The listing builds one solid part. Answer for the finished solid, in the listing's coordinates (mm). Face numbers are marked on the shaded views. A direction names the side the tool comes from. Give positions to 0.01 mm unless a question says otherwise; leave off trailing zeros. Write each loop counter-clockwise with the first axis right and the second up, starting at its lowest first coordinate (ties: lowest second). Pieces come first, ordered by that corner, then holes. Notation, with made-up numbers: (46, 20) - (80, 20) arc R26 ccw to (80, 37) - close; hole circle Ø11 at (86.25, 70). An arc over 180 degrees is marked (long way). Use a Markdown table: item, result. Add a question column.
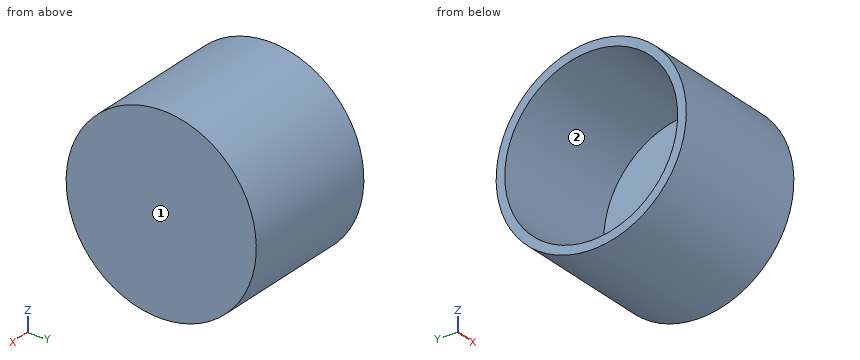
Autodesk Inventor part; units mm, degrees
ref_plane "YZ Plane" through (0, 0, 0) normal (1, 0, 0) x (0, 1, 0)
ref_plane "XZ Plane" through (0, 0, 0) normal (0, 1, 0) x (-1, 0, 0)
ref_plane "XY Plane" through (0, 0, 0) normal (0, 0, 1) x (1, 0, 0)
sketch "Sketch1" plane through (0, 0, 0) normal (1, 0, 0) x (0, 1, 0)
  circle A0 centre (0, 0) radius 4.191
  circle A1 centre (0, 0) radius 3.81
  dimension "d0" = 8.382
  dimension "d1" = 7.62
extrude "Extrusion1" add sketch "Sketch1" along normal blind 1.27
sketch "Sketch2" plane through (0, 0, 0) normal (-1, 0, 0) x (0, 0, 1)
  circle A0 centre (0, 0) radius 4.191
  circle A1 centre (0, 0) radius 3.81
  dimension "d5" = 8.382
  dimension "d4" = 7.62
extrude "Extrusion2" add sketch "Sketch2" along normal blind 1.27
sketch "Sketch3" plane through (-1.27, 0, 0) normal (-1, 0, 0) x (0, 0, 1)
  circle A0 centre (0, 0) radius 4.191
  circle A1 centre (0, 0) radius 3.81
  dimension "d10" = 8.382
  dimension "d9" = 7.62
extrude "Extrusion3" add sketch "Sketch3" along normal blind 1.27
sketch "Sketch4" plane through (1.27, 0, 0) normal (1, 0, 0) x (0, 0, -1)
  circle A0 centre (0, 0) radius 4.191
  circle A1 centre (0, 0) radius 3.81
  dimension "d15" = 8.382
  dimension "d14" = 7.62
extrude "Extrusion4" add sketch "Sketch4" along normal blind 1.27
sketch "Sketch5" plane through (2.54, 0, 0) normal (1, 0, 0) x (0, 0, -1)
  circle A0 centre (0, 0) radius 4.191
  circle A1 centre (0, 0) radius 3.81
  dimension "d20" = 8.382
  dimension "d19" = 7.62
extrude "Extrusion5" add sketch "Sketch5" along normal blind 1.27
sketch "Sketch6" plane through (3.81, 0, 0) normal (1, 0, 0) x (0, 0, -1)
  circle A0 centre (0, 0) radius 3.81
extrude "Extrusion6" add sketch "Sketch6" against normal blind 0.508
properties part number "rond"
1. The part is cut by section B-B (y = -1.25). Give the vertices of the cut face in (x, z), and give its area (3 significant figures).
2. The part is cut by section A-A (x = 1). Give the vertices of the cut face in (y, z).
3. The part is cut by section C-C (y = -3.5). Give the vertices of the cut face in (x, z).
4. Which of the six approach directions +Z, -Z, +X, -X, +Y, -Y give full straight-line access (tool end or side, diameter ignored) to the marked faces 1 and 2?
5. Consider L1, parallel to Z at x = 0.8, y = 0; L2, parallel to X at y = 3.25, z = -1.5. Determine where each line is inside the solid, lowest interval first. Write a range as [from, to].
6. Given P1, Ø1, axis at x = 0, z = -1.5, coming from the +Y side; P2, Ø4, axis at y = 0.5, z = -0.5, coming from the -X side; P3, Ø1, axis at x = 0, y = -1, coming from the +Z side, each flat-ended and moving along its own axis, determine where each tip first touches the part or whether it passes through.
Check values:
| question | item | result |
|---|---|---|
| 1 | outline | (-2.54, -4) - (3.81, -4) - (3.81, 4) - (-2.54, 4) - (-2.54, 3.6) - (3.3, 3.6) - (3.3, -3.6) - (-2.54, -3.6) - close |
| 1 | area | 8.75 mm2 |
| 2 | outline | circle Ø8.38 at (0, 0); hole circle Ø7.62 at (0, 0) |
| 3 | outline | (-2.54, -2.31) - (3.81, -2.31) - (3.81, 2.31) - (-2.54, 2.31) - (-2.54, 1.51) - (3.3, 1.51) - (3.3, -1.51) - (-2.54, -1.51) - close |
| 4 | face 1 | +Z, -Z, +X, +Y, -Y |
| 4 | face 2 | -X |
| 5 | L1 | z = [-4.19, -3.81], [3.81, 4.19] |
| 5 | L2 | x = [3.3, 3.81] |
| 6 | P1 | stops at y = 4.07 |
| 6 | P2 | stops at x = 3.3 |
| 6 | P3 | stops at z = 4.16 |
